from build123d import *

# Parameters (mm, degrees)
BOSS_EXTRUDE1_DEPTH    = 3.175
F_10_CLEARANCE_HOLE1_D = 5.1054


with BuildPart() as part:
    # Sketch1 → Boss-Extrude1 (new body)
    with BuildSketch(Plane(origin=(0, 0, 0), x_dir=(1, 0, 0), z_dir=(0, 1, 0))):
        with BuildLine():
            Line((22.225, -19.05), (-22.225, -19.05))
            ThreePointArc((-22.225, -19.05), (-26.715128061, -17.190128061), (-28.575, -12.7))
            Line((-28.575, -12.7), (-28.575, 12.7))
            ThreePointArc((-28.575, 12.7), (-26.715128061, 17.190128061), (-22.225, 19.05))
            Line((-22.225, 19.05), (22.225, 19.05))
            ThreePointArc((22.225, 19.05), (26.715128061, 17.190128061), (28.575, 12.7))
            Line((28.575, 12.7), (28.575, -12.7))
            ThreePointArc((28.575, -12.7), (26.715128061, -17.190128061), (22.225, -19.05))
        make_face()
    extrude(amount=BOSS_EXTRUDE1_DEPTH)

    # #10 Clearance Hole1 (through all)
    with Locations(Plane(origin=(0, 3.175, 0), x_dir=(1, 0, 0), z_dir=(0, 1, 0))):
        with Locations((-22.225, 12.7), (0, 12.7), (22.225, 12.7), (0, -12.7), (22.225, -12.7), (-22.225, -12.7)):
            Hole(F_10_CLEARANCE_HOLE1_D / 2)


solid = part.part
Read the model definition and answer for the solid it produces. Units are mm, in the model's axes. Round coordinates to 2 decimals unless told otherwise and drop trailing zeros. Write each loop counter-clockwise with the first axis right and the second up, starting at its lowest first coordinate (ties: lowest second). Pieces come first, ordered by that corner, then holes. Notation, with made-up numbers: M -37,85 L 4,85 A22 cw 4,98 Z; hole C 46,46 d2. An arc over 180 degrees is marked long. Use a Markdown table: item, result.
1) Straight lines are drawn through the part: line 1 along X through (y, z) = (2.35, -12.7) (3 decimals); line 2 along X through (y, z) = (2.7, -13); line 3 along Z through (x, y) = (-21, 2.9). For each, find the intervals that lie inside material, in ascending order. Write a range as [from, to].
Answers follow:
| item | result |
|---|---|
| line 1 | x = [-28.575, -24.778], [-19.672, -2.553], [2.553, 19.672], [24.778, 28.575] |
| line 2 | x = [-28.57, -24.76], [-19.69, -2.54], [2.54, 19.69], [24.76, 28.57] |
| line 3 | z = [-19.05, -14.94], [-10.46, 10.46], [14.94, 19.05] |
2) The part is cut by section D-D (x = 23.5). Write down the section's boundary in (y, z) (3 decimals).
Answers follow:
| item | result |
|---|---|
| outline | M 0,-18.921 L 3.175,-18.921 L 3.175,-14.911 L 0,-14.911 Z; M 0,-10.489 L 3.175,-10.489 L 3.175,10.489 L 0,10.489 Z; M 0,14.911 L 3.175,14.911 L 3.175,18.921 L 0,18.921 Z |
3) The part is cut by section C-C (y = 0.7). Write down the section's boundary in (x, z) (3 decimals).
Answers follow:
| item | result |
|---|---|
| outline | M -28.575,-12.7 A6.35 ccw -22.225,-19.05 L 22.225,-19.05 A6.35 ccw 28.575,-12.7 L 28.575,12.7 A6.35 ccw 22.225,19.05 L -22.225,19.05 A6.35 ccw -28.575,12.7 Z; hole C -22.225,-12.7 d5.105; hole C -22.225,12.7 d5.105; hole C 0,-12.7 d5.105; hole C 0,12.7 d5.105; hole C 22.225,-12.7 d5.105; hole C 22.225,12.7 d5.105 |
4) The part is cut by section B-B (z = 11). Write down the section's boundary in (x, y) (3 decimals), plus the area to 3 significant figures.
Answers follow:
| item | result |
|---|---|
| outline | M -28.575,0 L -24.129,0 L -24.129,3.175 L -28.575,3.175 Z; M -20.321,0 L -1.904,0 L -1.904,3.175 L -20.321,3.175 Z; M 1.904,0 L 20.321,0 L 20.321,3.175 L 1.904,3.175 Z; M 24.129,0 L 28.575,0 L 28.575,3.175 L 24.129,3.175 Z |
| area | 145 mm2 |
5) For a pull along X with two mould halves and no side action, classify faces 1 (the cylindrical face through (0.553, 1.565, 15.192)), 2 (the cylindrical face through (-26.764, 1.565, -17.14)), 3 (the flat face through (0, 0, 0)), 4 (the cylindrical face through (0.553, 1.565, -10.208)) as pulls with the +X half, pulls with the -X half, needs draft (parallel to the pull), parting line crosses it, or undercut.
Answers follow:
| item | result |
|---|---|
| face 1 | undercut |
| face 2 | pulls with the -X half |
| face 3 | needs draft |
| face 4 | undercut |
6) The part is cut by section A-A (x = 0). Write down the section's boundary in (y, z) (3 decimals).
Answers follow:
| item | result |
|---|---|
| outline | M 0,-19.05 L 3.175,-19.05 L 3.175,-15.253 L 0,-15.253 Z; M 0,-10.147 L 3.175,-10.147 L 3.175,10.147 L 0,10.147 Z; M 0,15.253 L 3.175,15.253 L 3.175,19.05 L 0,19.05 Z |
